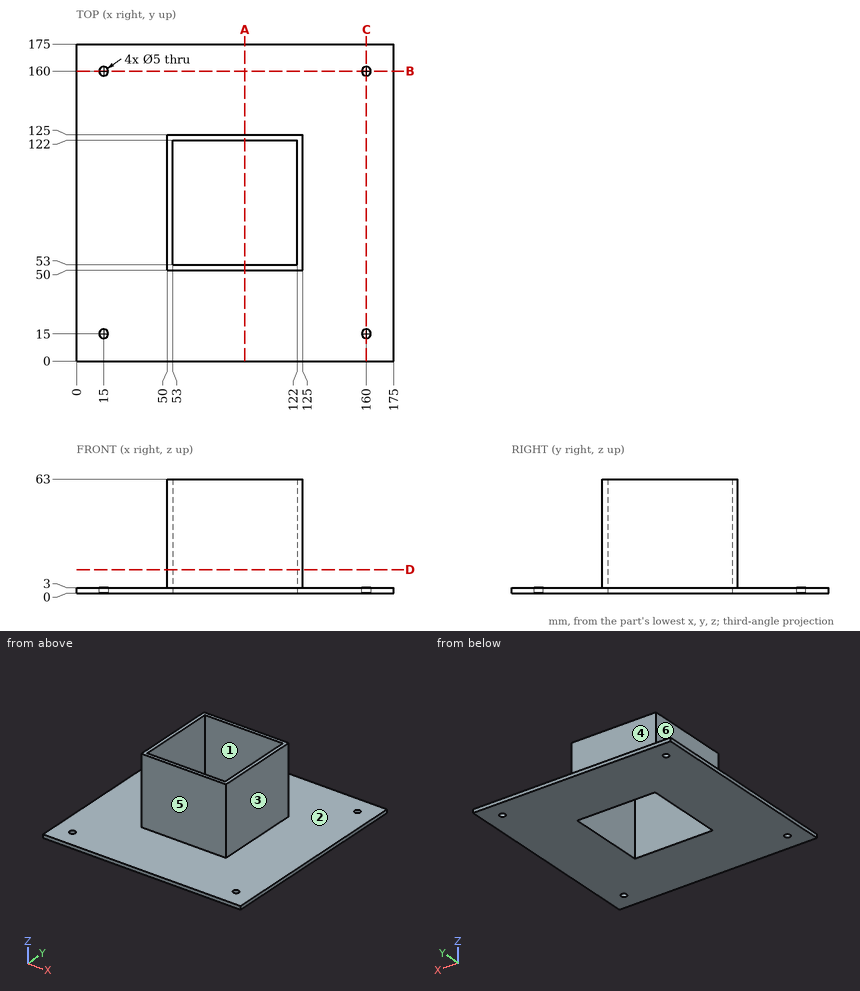
Geometry: see drawing. Coordinates: mm, zero at the bounding-box minimum. A direction names the side the tool comes from. Round coordinates to 2 decimals unless told otherwise and drop trailing zeros. Loops run counter-clockwise (first coordinate to the right, second up) from the corner with the lowest first, then second, coordinate; pieces in that order, holes last. Notation, with made-up numbers: (-39, 1) - (-27, 1) arc R15 ccw to (-27, 23) - close; hole circle Ø9 at (-3.75, -12.75). An arc over 180 degrees is marked (long way). Write item = value, one per line. Start each with the question number.
(1) Set-up query: the marked faces 4, 5 and 6. Return all of +Z, -Z, +X, -X, +Y, -Y with unobstructed straight access to the full face (end or side cutting, diameter ignored); none if empty.
(2) Section query D-D, the plane z = 13. Output: boundary loops of the cut face in (x, y).
(3) Pin query (flat end, axial travel): pin 1 (8 mm diameter, centred on x = 30, y = 111, fed in from +Z); pin 2 (1 mm diameter, centred on y = 89.5, z = 19.5, fed in from +X); pin 3 (2 mm diameter, centred on y = 93.5, z = 28, fed in from -X). Return the tip coordinate at first contact, or that it passes through.
(4) Pull-direction query (X, two-part tool) for the marked faces 1, 2 and 3; classes: +X half, -X half, draft (parallel to the pull), parting line (faces both ways), or undercut.
(5) Ray query, line 1 along Y through (x, z) = (15, 1); line 2 along X through (y, z) = (70.5, 56.5). Return the intervals inside material, ascending. Write a range as from..to.
(6) Section query B-B, the plane y = 160. Output: boundary loops of the cut face in (x, z), plus the area to 3 significant figures.
(7) Section query A-A, the plane x = 93. Output: boundary loops of the cut face in (y, z), plus the area to 3 significant figures.
Conclusion:
q1.face_4 = +Z, +X, -X, +Y
q1.face_5 = +Z, +X, -X, -Y
q1.face_6 = +Z, -X, +Y, -Y
q2.outline = (50, 50) - (125, 50) - (125, 125) - (50, 125) - close; hole (53, 53) - (122, 53) - (122, 122) - (53, 122) - close
q3.pin_1 = 3
q3.pin_2 = 125
q3.pin_3 = 50
q4.face_1 = undercut
q4.face_2 = draft
q4.face_3 = +X half
q5.line_1 = 0..12.5, 17.5..157.5, 162.5..175
q5.line_2 = 50..53, 122..125
q6.outline = (0, 0) - (12.5, 0) - (12.5, 3) - (0, 3) - close; (17.5, 0) - (157.5, 0) - (157.5, 3) - (17.5, 3) - close; (162.5, 0) - (175, 0) - (175, 3) - (162.5, 3) - close
q6.area = 495 mm2
q7.outline = (0, 0) - (53, 0) - (53, 63) - (50, 63) - (50, 3) - (0, 3) - close; (122, 0) - (175, 0) - (175, 3) - (125, 3) - (125, 63) - (122, 63) - close
q7.area = 678 mm2
